```python
from build123d import *

# Parameters (mm, degrees)
SKETCH1_R           = 10
BOSS_EXTRUDE1_DEPTH = 12
FILLET1_R           = 0.5
SKETCH2_R           = 3
CUT_EXTRUDE1_DEPTH  = 10
BOSS_EXTRUDE2_DEPTH = 0.01


with BuildPart() as part:
    # Sketch1 → Boss-Extrude1 (new body)
    with BuildSketch(Plane(origin=(0, 0, 0), x_dir=(1, 0, 0), z_dir=(0, 1, 0))):
        Circle(SKETCH1_R)
    extrude(amount=BOSS_EXTRUDE1_DEPTH)

    # Fillet1
    fillet1_edges = [part.edges().sort_by_distance(p)[0] for p in [
        (-10, 12, 0),
    ]]
    fillet(fillet1_edges, radius=FILLET1_R)

    # Sketch2 → Cut-Extrude1 (cut)
    with BuildSketch(Plane.XZ):
        Circle(SKETCH2_R)
    extrude(amount=-CUT_EXTRUDE1_DEPTH, mode=Mode.SUBTRACT)

    # Sketch3 → Boss-Extrude2 (add)
    with BuildSketch(Plane(origin=(0, 12, 0), x_dir=(1, 0, 0), z_dir=(0, 1, 0))):
        Polygon((-7, -1), (-7, 1), (-9, 0), align=None)
    extrude(amount=BOSS_EXTRUDE2_DEPTH)


solid = part.part
```
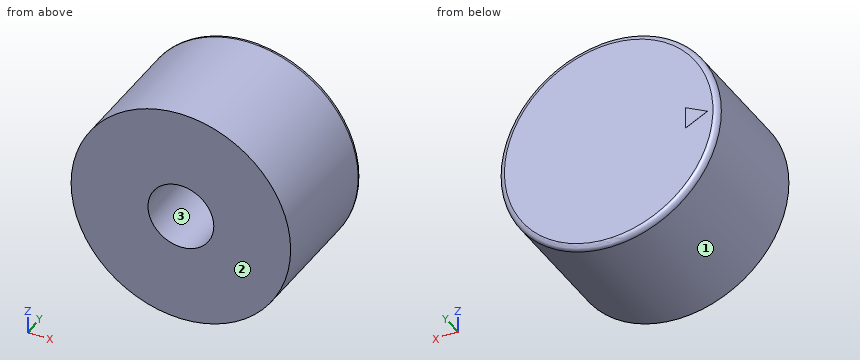
Source: CAD feature listing. Evaluate the final solid. Frame: model axes, mm. Face numbers are marked on the shaded views. Coordinates: 2 decimals unless noted, no trailing zeros. Loops run counter-clockwise (first coordinate to the right, second up) from the corner with the lowest first, then second, coordinate; pieces in that order, holes last. Notation, with made-up numbers: (-13.5, -18.75) -> (38.5, -18.75) arc R16 ccw to (38.5, -6.75) -> close; hole circle Ø7 at (52, 73). An arc over 180 degrees is marked (long way). One line per item, written item: value. Start each with the question number.
Q1. Section query B-B, the plane y = 3.5. Return the cut outline in (x, z), and give its area (3 significant figures).
Q2. Line query: line 1 along Y through (x, z) = (-4.25, 2.25); line 2 along Z through (x, y) = (0, 3.25); line 3 along X through (y, z) = (2.5, -0.25). Output: solid intervals per line, ascending.
Q3. Section query A-A, the plane x = 0. Return the cut outline in (y, z), and give its area (3 significant figures).
Q4. Mould query, pull axis Z, two halves, no side actions, for the marked faces 1, 2 and 3. Classes: pulls with the +Z half, pulls with the -Z half, needs draft (parallel to the pull), parting line crosses it, or undercut.
Q5. Contact query for flat-ended pins moving along their axis: P1, Ø1.5, axis at y = 7, z = 6, coming from the +X side; P2, Ø6, axis at x = 1.5, z = 5, coming from the +Y side; P3, Ø1.5, axis at x = -2, y = 2, coming from the +Z side. Output: stop coordinate, or through.
Results:
1. outline: circle Ø20 at (0, 0); hole circle Ø6 at (0, 0)
1. area: 286 mm^2
2. line 1: 0 to 12
2. line 2: -10 to -3, 3 to 10
2. line 3: -10 to -2.99, 2.99 to 10
3. outline: (0, -10) -> (11.5, -10) arc R0.5 ccw to (12, -9.5) -> (12, 9.5) arc R0.5 ccw to (11.5, 10) -> (0, 10) -> (0, 3) -> (10, 3) -> (10, -3) -> (0, -3) -> close
3. area: 180 mm^2
4. face 1: parting line crosses it
4. face 2: needs draft
4. face 3: undercut
5. P1: x = 8.51
5. P2: y = 12
5. P3: z = 9.92
